from build123d import *

# Parameters (mm, degrees)
SKETCH1_W           = 177.8
SKETCH1_H           = 50.8
SKETCH1_R           = 8.73125
SKETCH1_R_2         = 1.8288
BOSS_EXTRUDE1_DEPTH = 6.35


with BuildPart() as part:
    # Sketch1 → Boss-Extrude1 (new body)
    with BuildSketch(Plane.XY):
        with Locations((0, -10.31875)):
            Rectangle(SKETCH1_W, SKETCH1_H)
        Circle(SKETCH1_R, mode=Mode.SUBTRACT)
        with Locations((-79.0575, 0)):
            Circle(SKETCH1_R_2, mode=Mode.SUBTRACT)
        with Locations((-60.6425, 0)):
            Circle(SKETCH1_R_2, mode=Mode.SUBTRACT)
        with Locations((60.6425, 0)):
            Circle(SKETCH1_R_2, mode=Mode.SUBTRACT)
        with Locations((79.0575, 0)):
            Circle(SKETCH1_R_2, mode=Mode.SUBTRACT)
        with Locations((69.85, 9.2075)):
            Circle(SKETCH1_R_2, mode=Mode.SUBTRACT)
        with Locations((69.85, -9.2075)):
            Circle(SKETCH1_R_2, mode=Mode.SUBTRACT)
        with Locations((-69.85, 9.2075)):
            Circle(SKETCH1_R_2, mode=Mode.SUBTRACT)
        with Locations((-69.85, -9.2075)):
            Circle(SKETCH1_R_2, mode=Mode.SUBTRACT)
        with Locations((-76.2, -19.84375)):
            Circle(SKETCH1_R_2, mode=Mode.SUBTRACT)
        with Locations((-63.5, -19.84375)):
            Circle(SKETCH1_R_2, mode=Mode.SUBTRACT)
        with Locations((-63.5, -32.54375)):
            Circle(SKETCH1_R_2, mode=Mode.SUBTRACT)
        with Locations((-76.2, -32.54375)):
            Circle(SKETCH1_R_2, mode=Mode.SUBTRACT)
        with Locations((63.5, -19.84375)):
            Circle(SKETCH1_R_2, mode=Mode.SUBTRACT)
        with Locations((76.2, -19.84375)):
            Circle(SKETCH1_R_2, mode=Mode.SUBTRACT)
        with Locations((76.2, -32.54375)):
            Circle(SKETCH1_R_2, mode=Mode.SUBTRACT)
        with Locations((63.5, -32.54375)):
            Circle(SKETCH1_R_2, mode=Mode.SUBTRACT)
    extrude(amount=BOSS_EXTRUDE1_DEPTH)


solid = part.part
Design review of the part built by this model. Coordinates are the model's own, in mm. Give positions to 0.01 mm unless a question says otherwise; leave off trailing zeros. Write each loop counter-clockwise with the first axis right and the second up, starting at its lowest first coordinate (ties: lowest second). Pieces come first, ordered by that corner, then holes. Notation, with made-up numbers: M -38.75,-30 L 4.25,-30 A22 ccw 4.25,-14 Z; hole C -15,-20.75 d4. An arc over 180 degrees is marked long. Answer as a JSON object with one key per item and string values. Group by question number.
1) For line 1 along X through (y, z) = (9.5, 2.5); line 2 along Y through (x, z) = (-63.5, 2); line 3 along X through (y, z) = (-20, 1), list the stretches that pass through material, from the lowest coordinate up.
2) We need section C-C (z = 2). Count the separate pieces of the cut face and the enclosed holes in it, and give its area (3 significant figures).
3) Clearance check with flat-ended pins moving along their axes: pin 1 Ø4 at (x, y) = (76.2, -32.54) entering from -Z; pin 2 Ø3.5 at (x, y) = (-60.64, 0) entering from -Z. State where each tip first meets the part, or that it passes through.
4) Mouldability with a two-part tool opening along Y and no side actions: class faces 1 (the face through (-74.456, -19.294, 3.131)), 2 (the face through (-1, 15.081, 3)), 3 (the face through (-1, -10, 0)) as released by +Y, released by -Y, zero draft, split by the parting line, or undercut.
5) We need section A-A (x = 69.85). Give the boundary of the cut face in (y, z), and give its area (3 significant figures).
6) We need section B-B (x = 0). Give the boundary of the cut face in (y, z), and give its area (3 significant figures).
Answer key:
{
 "1": {"line 1": "x = -88.9 to -71.66, -68.04 to 68.04, 71.66 to 88.9", "line 2": "y = -35.72 to -34.37, -30.71 to -21.67, -18.01 to 15.08", "line 3": "x = -88.9 to -78.02, -74.38 to -65.32, -61.68 to 61.68, 65.32 to 74.38, 78.02 to 88.9"},
 "2": {"separate pieces": "1", "enclosed holes": "17", "area": "8,620 mm²"},
 "3": {"pin 1": "stops at z = 0", "pin 2": "passes through"},
 "4": {"face 1": "undercut", "face 2": "released by +Y", "face 3": "zero draft"},
 "5": {"outline": "M -35.72,0 L -11.04,0 L -11.04,6.35 L -35.72,6.35 Z; M -7.38,0 L 7.38,0 L 7.38,6.35 L -7.38,6.35 Z; M 11.04,0 L 15.08,0 L 15.08,6.35 L 11.04,6.35 Z", "area": "276 mm²"},
 "6": {"outline": "M -35.72,0 L -8.73,0 L -8.73,6.35 L -35.72,6.35 Z; M 8.73,0 L 15.08,0 L 15.08,6.35 L 8.73,6.35 Z", "area": "212 mm²"}
}
